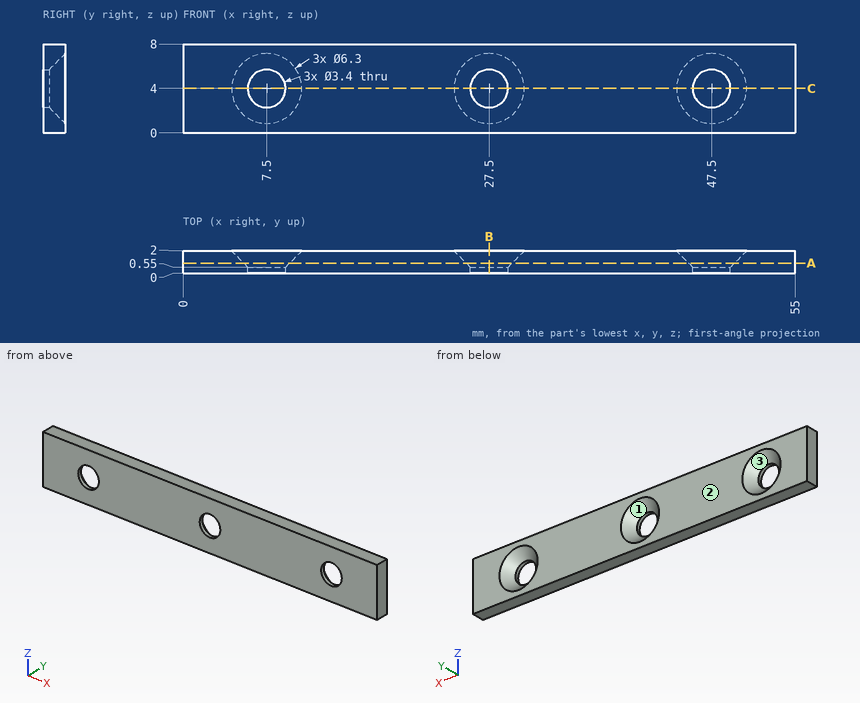
Could you check a few things on this drawing? It's one solid part, dimensions in mm from its lowest x, y, z. Give positions to 0.01 mm unless a question says otherwise; leave off trailing zeros. Order: outer loops, then holes, each group sorted by start corner. A loop starts at its lowest first (then second) coordinate and runs counter-clockwise, first axis right, second up.
1. Thinking about a two-plate mould opening in Z: for the marked faces 1, 2 and 3, which applies, +Z half, -Z half, draft (parallel to the pull), parting line (faces both ways), or undercut?
Answers below:
face 1: undercut
face 2: draft
face 3: undercut
2. Suppose I cut it at C-C (z = 4). Write out the boundary of the cut face in (x, y).
Answers below:
outline: (0, 0) - (5.8, 0) - (5.8, 0.55) - (4.35, 2) - (0, 2) - close; (9.2, 0) - (25.8, 0) - (25.8, 0.55) - (24.35, 2) - (10.65, 2) - (9.2, 0.55) - close; (29.2, 0) - (45.8, 0) - (45.8, 0.55) - (44.35, 2) - (30.65, 2) - (29.2, 0.55) - close; (49.2, 0) - (55, 0) - (55, 2) - (50.65, 2) - (49.2, 0.55) - close
3. I need wall thicknesses on L1, parallel to X at y = 0.3, z = 4; L2, parallel to Z at x = 7.5, y = 0.4; L3, parallel to X at y = 1.6, z = 6. Which ranges of each line are inside material? Lowest first, please.
Answers below:
L1: x = 0 to 5.8, 9.2 to 25.8, 29.2 to 45.8, 49.2 to 55
L2: z = 0 to 2.3, 5.7 to 8
L3: x = 0 to 5.61, 9.39 to 25.61, 29.39 to 45.61, 49.39 to 55
4. Suppose I cut it at B-B (x = 27.5). Write out the boundary of the cut face in (y, z).
Answers below:
outline: (0, 0) - (2, 0) - (2, 0.85) - (0.55, 2.3) - (0, 2.3) - close; (0, 5.7) - (0.55, 5.7) - (2, 7.15) - (2, 8) - (0, 8) - close
5. Suppose I cut it at A-A (y = 0.9). Write out the boundary of the cut face in (x, z).
Answers below:
outline: (0, 0) - (55, 0) - (55, 8) - (0, 8) - close; hole circle Ø4.1 at (7.5, 4); hole circle Ø4.1 at (27.5, 4); hole circle Ø4.1 at (47.5, 4)
